Here's how the part is built. I have some questions about the finished solid (model axes, mm). Give positions to 0.01 mm unless a question says otherwise; leave off trailing zeros. Loops run counter-clockwise (first coordinate to the right, second up) from the corner with the lowest first, then second, coordinate; pieces in that order, holes last. Notation, with made-up numbers: (71, 60) - (93, 60) arc R22 cw to (93, 82) - close; hole circle Ø1 at (-33, 70.5). An arc over 180 degrees is marked (long way). Use a Markdown table: item, result.
from build123d import *
from OCP.BRepFilletAPI import BRepFilletAPI_MakeChamfer

# Parameters (mm, degrees)
SKETCH1_W                     = 2.54
SKETCH1_H                     = 2.54
MAIN_BODY_DEPTH               = 2.54
SKETCH3_W                     = 1.778
SKETCH3_H                     = 0.381
CUT_EXTRUDE1_DEPTH            = 5.399409051
CUT_EXTRUDE2_DEPTH            = 5.399409051
BODY_PATTERN_COUNT            = 3
BODY_PATTERN_PITCH            = 2.54
PIN_START                     = -5.54
SKETCH2_W                     = 0.64
SKETCH2_H                     = 0.64
PIN_DEPTH                     = 11.54
CHAMFER1_SIZE                 = 0.508
CHAMFER1_SIZE2                = 0.1905
CHAMFER2_SIZE                 = 0.1905
CHAMFER2_SIZE2                = 0.508
PIN_PATTERN_COUNT             = 3
PIN_PATTERN_PITCH             = 2.54
CHAMFER1_OF_PIN_PATTERN_SIZE  = 0.508
CHAMFER1_OF_PIN_PATTERN_SIZE2 = 0.1905
CHAMFER2_OF_PIN_PATTERN_SIZE2 = 0.1905
CHAMFER2_OF_PIN_PATTERN_SIZE  = 0.508


with BuildPart() as part:
    # Sketch1 → Main Body (new body)
    with BuildSketch(Plane(origin=(0, 0, 0), x_dir=(1, 0, 0), z_dir=(0, 1, 0))):
        with Locations((1.27, 1.27)):
            Rectangle(SKETCH1_W, SKETCH1_H)
    main_body = extrude(amount=MAIN_BODY_DEPTH)

    # Sketch3 → Cut-Extrude1 (cut, through all)
    with BuildSketch(Plane.ZY):
        with Locations((-1.27, 0.1905)):
            Rectangle(SKETCH3_W, SKETCH3_H)
    cut_extrude1 = extrude(amount=-CUT_EXTRUDE1_DEPTH, mode=Mode.SUBTRACT)

    # Sketch4 → Cut-Extrude2 (cut, through all)
    with BuildSketch(Plane(origin=(0, 2.54, 0), x_dir=(1, 0, 0), z_dir=(0, 1, 0))):
        Polygon((0.254, 2.54), (0, 2.54), (0, 2.032), align=None)
        Polygon((2.54, 2.54), (2.286, 2.54), (2.54, 2.032), align=None)
        Polygon((0.254, 0), (0, 0.508), (0, 0), align=None)
        Polygon((2.54, 0), (2.286, 0), (2.54, 0.508), align=None)
    cut_extrude2 = extrude(amount=-CUT_EXTRUDE2_DEPTH, mode=Mode.SUBTRACT)

    # Body Pattern: Main Body, Cut-Extrude1, Cut-Extrude2 ×3
    with Locations(*[(-i * BODY_PATTERN_PITCH, 0, 0) for i in range(1, BODY_PATTERN_COUNT)]):
        add(main_body)
        add(cut_extrude1, mode=Mode.SUBTRACT)
        add(cut_extrude2, mode=Mode.SUBTRACT)

    # Sketch2 → Pin (add)
    with BuildSketch(Plane(origin=(0, 2.54, 0), x_dir=(1, 0, 0), z_dir=(0, 1, 0)).offset(PIN_START)):
        with Locations((1.27, 1.27)):
            Rectangle(SKETCH2_W, SKETCH2_H)
    pin = extrude(amount=PIN_DEPTH)

    # Chamfer1: one chamfer whose edges measure the first distance from different faces: ONE call of the kernel's chamfer builder (chamfer() names one face for all edges)
    chamfer1_edges_1 = [part.edges().sort_by_distance(p)[0] for p in [
        (0.95, 8.54, -1.27),
    ]]
    chamfer1_side_1 = [part.faces().sort_by_distance(p)[0] for p in [
        (0.95, 5.54, -1.27),
    ]]
    chamfer1_edges_2 = [part.edges().sort_by_distance(p)[0] for p in [
        (1.27, 8.54, -0.95),
    ]]
    chamfer1_side_2 = [part.faces().sort_by_distance(p)[0] for p in [
        (1.27, 5.54, -0.95),
    ]]
    chamfer1_edges_3 = [part.edges().sort_by_distance(p)[0] for p in [
        (1.59, 8.54, -1.27),
    ]]
    chamfer1_side_3 = [part.faces().sort_by_distance(p)[0] for p in [
        (1.59, 5.54, -1.27),
    ]]
    chamfer1_edges_4 = [part.edges().sort_by_distance(p)[0] for p in [
        (1.27, 8.54, -1.59),
    ]]
    chamfer1_side_4 = [part.faces().sort_by_distance(p)[0] for p in [
        (1.27, 5.54, -1.59),
    ]]
    chamfer1 = BRepFilletAPI_MakeChamfer(part.part.solid().wrapped)
    for e in chamfer1_edges_1:
        chamfer1.Add(CHAMFER1_SIZE, CHAMFER1_SIZE2, e.wrapped, chamfer1_side_1[0].wrapped)  # the first distance lies on this face
    for e in chamfer1_edges_2:
        chamfer1.Add(CHAMFER1_SIZE, CHAMFER1_SIZE2, e.wrapped, chamfer1_side_2[0].wrapped)  # the first distance lies on this face
    for e in chamfer1_edges_3:
        chamfer1.Add(CHAMFER1_SIZE, CHAMFER1_SIZE2, e.wrapped, chamfer1_side_3[0].wrapped)  # the first distance lies on this face
    for e in chamfer1_edges_4:
        chamfer1.Add(CHAMFER1_SIZE, CHAMFER1_SIZE2, e.wrapped, chamfer1_side_4[0].wrapped)  # the first distance lies on this face
    add(Compound.cast(chamfer1.Shape()), mode=Mode.REPLACE)

    # Chamfer2
    chamfer2_edges = [part.edges().sort_by_distance(p)[0] for p in [
        (1.27, -3, -0.95),
        (1.59, -3, -1.27),
        (1.27, -3, -1.59),
        (0.95, -3, -1.27),
    ]]
    chamfer2_side = [part.faces().sort_by_distance(p)[0] for p in [
        (1.27, -3, -1.27),
    ]]
    chamfer(chamfer2_edges, length=CHAMFER2_SIZE, length2=CHAMFER2_SIZE2, reference=chamfer2_side[0])

    # Pin Pattern: Pin ×3
    with Locations(*[(-i * PIN_PATTERN_PITCH, 0, 0) for i in range(1, PIN_PATTERN_COUNT)]):
        add(pin)

    # Chamfer1 of Pin Pattern: one chamfer whose edges measure the first distance from different faces: ONE call of the kernel's chamfer builder (chamfer() names one face for all edges)
    chamfer1_of_pin_pattern_edges_1 = [part.edges().sort_by_distance(p)[0] for p in [
        (-1.59, 8.54, -1.27),
    ]]
    chamfer1_of_pin_pattern_side_1 = [part.faces().sort_by_distance(p)[0] for p in [
        (-1.59, 5.54, -1.27),
    ]]
    chamfer1_of_pin_pattern_edges_2 = [part.edges().sort_by_distance(p)[0] for p in [
        (-1.27, 8.54, -0.95),
    ]]
    chamfer1_of_pin_pattern_side_2 = [part.faces().sort_by_distance(p)[0] for p in [
        (-1.27, 5.54, -0.95),
    ]]
    chamfer1_of_pin_pattern_edges_3 = [part.edges().sort_by_distance(p)[0] for p in [
        (-0.95, 8.54, -1.27),
    ]]
    chamfer1_of_pin_pattern_side_3 = [part.faces().sort_by_distance(p)[0] for p in [
        (-0.95, 5.54, -1.27),
    ]]
    chamfer1_of_pin_pattern_edges_4 = [part.edges().sort_by_distance(p)[0] for p in [
        (-1.27, 8.54, -1.59),
    ]]
    chamfer1_of_pin_pattern_side_4 = [part.faces().sort_by_distance(p)[0] for p in [
        (-1.27, 5.54, -1.59),
    ]]
    chamfer1_of_pin_pattern_edges_5 = [part.edges().sort_by_distance(p)[0] for p in [
        (-4.13, 8.54, -1.27),
    ]]
    chamfer1_of_pin_pattern_side_5 = [part.faces().sort_by_distance(p)[0] for p in [
        (-4.13, 5.54, -1.27),
    ]]
    chamfer1_of_pin_pattern_edges_6 = [part.edges().sort_by_distance(p)[0] for p in [
        (-3.81, 8.54, -0.95),
    ]]
    chamfer1_of_pin_pattern_side_6 = [part.faces().sort_by_distance(p)[0] for p in [
        (-3.81, 5.54, -0.95),
    ]]
    chamfer1_of_pin_pattern_edges_7 = [part.edges().sort_by_distance(p)[0] for p in [
        (-3.49, 8.54, -1.27),
    ]]
    chamfer1_of_pin_pattern_side_7 = [part.faces().sort_by_distance(p)[0] for p in [
        (-3.49, 5.54, -1.27),
    ]]
    chamfer1_of_pin_pattern_edges_8 = [part.edges().sort_by_distance(p)[0] for p in [
        (-3.81, 8.54, -1.59),
    ]]
    chamfer1_of_pin_pattern_side_8 = [part.faces().sort_by_distance(p)[0] for p in [
        (-3.81, 5.54, -1.59),
    ]]
    chamfer1_of_pin_pattern = BRepFilletAPI_MakeChamfer(part.part.solid().wrapped)
    for e in chamfer1_of_pin_pattern_edges_1:
        chamfer1_of_pin_pattern.Add(CHAMFER1_OF_PIN_PATTERN_SIZE, CHAMFER1_OF_PIN_PATTERN_SIZE2, e.wrapped, chamfer1_of_pin_pattern_side_1[0].wrapped)  # the first distance lies on this face
    for e in chamfer1_of_pin_pattern_edges_2:
        chamfer1_of_pin_pattern.Add(CHAMFER1_OF_PIN_PATTERN_SIZE, CHAMFER1_OF_PIN_PATTERN_SIZE2, e.wrapped, chamfer1_of_pin_pattern_side_2[0].wrapped)  # the first distance lies on this face
    for e in chamfer1_of_pin_pattern_edges_3:
        chamfer1_of_pin_pattern.Add(CHAMFER1_OF_PIN_PATTERN_SIZE, CHAMFER1_OF_PIN_PATTERN_SIZE2, e.wrapped, chamfer1_of_pin_pattern_side_3[0].wrapped)  # the first distance lies on this face
    for e in chamfer1_of_pin_pattern_edges_4:
        chamfer1_of_pin_pattern.Add(CHAMFER1_OF_PIN_PATTERN_SIZE, CHAMFER1_OF_PIN_PATTERN_SIZE2, e.wrapped, chamfer1_of_pin_pattern_side_4[0].wrapped)  # the first distance lies on this face
    for e in chamfer1_of_pin_pattern_edges_5:
        chamfer1_of_pin_pattern.Add(CHAMFER1_OF_PIN_PATTERN_SIZE, CHAMFER1_OF_PIN_PATTERN_SIZE2, e.wrapped, chamfer1_of_pin_pattern_side_5[0].wrapped)  # the first distance lies on this face
    for e in chamfer1_of_pin_pattern_edges_6:
        chamfer1_of_pin_pattern.Add(CHAMFER1_OF_PIN_PATTERN_SIZE, CHAMFER1_OF_PIN_PATTERN_SIZE2, e.wrapped, chamfer1_of_pin_pattern_side_6[0].wrapped)  # the first distance lies on this face
    for e in chamfer1_of_pin_pattern_edges_7:
        chamfer1_of_pin_pattern.Add(CHAMFER1_OF_PIN_PATTERN_SIZE, CHAMFER1_OF_PIN_PATTERN_SIZE2, e.wrapped, chamfer1_of_pin_pattern_side_7[0].wrapped)  # the first distance lies on this face
    for e in chamfer1_of_pin_pattern_edges_8:
        chamfer1_of_pin_pattern.Add(CHAMFER1_OF_PIN_PATTERN_SIZE, CHAMFER1_OF_PIN_PATTERN_SIZE2, e.wrapped, chamfer1_of_pin_pattern_side_8[0].wrapped)  # the first distance lies on this face
    add(Compound.cast(chamfer1_of_pin_pattern.Shape()), mode=Mode.REPLACE)

    # Chamfer2 of Pin Pattern
    chamfer2_of_pin_pattern_edges = [part.edges().sort_by_distance(p)[0] for p in [
        (-1.27, -3, -0.95),
        (-0.95, -3, -1.27),
        (-1.27, -3, -1.59),
        (-1.59, -3, -1.27),
        (-3.81, -3, -0.95),
        (-3.49, -3, -1.27),
        (-3.81, -3, -1.59),
        (-4.13, -3, -1.27),
    ]]
    chamfer(chamfer2_of_pin_pattern_edges, length=CHAMFER2_OF_PIN_PATTERN_SIZE, length2=CHAMFER2_OF_PIN_PATTERN_SIZE2)


solid = part.part
(1) If I drill on line 1 (X direction, y = 6.75, z = -1.2); line 2 (Z direction, x = 1, y = 0.25); line 3 (Z direction, x = -1.5, y = 5), over which ranges is the centre line in solid material (lowest first)?
A:
| item | result |
|---|---|
| line 1 | -4.13 to -3.49, -1.59 to -0.95, 0.95 to 1.59 |
| line 2 | -2.54 to -2.16, -1.59 to -0.95, -0.38 to 0 |
| line 3 | -1.59 to -0.95 |
(2) We'd pull the mould along X, two halves only. Please class faces 1 (the face through (-5.08, 1, -1)), 2 (the face through (-1, 0.381, -2)), 3 (the face through (-1, 1, 0)): pulls with the +X half, pulls with the -X half, needs draft (parallel to the pull), parting line crosses it, or undercut.
A:
| item | result |
|---|---|
| face 1 | pulls with the -X half |
| face 2 | undercut |
| face 3 | needs draft |
(3) Suppose I cut it at B-B on z = -0.2. Write out the boundary of the cut face in (x, y), plus the area to 3 significant figures.
A:
| item | result |
|---|---|
| outline | (-4.93, 0) - (-2.69, 0) - (-2.69, 2.54) - (-4.93, 2.54) - close; (-2.39, 0) - (-0.15, 0) - (-0.15, 2.54) - (-2.39, 2.54) - close; (0.15, 0) - (2.39, 0) - (2.39, 2.54) - (0.15, 2.54) - close |
| area | 17.0 mm2 |
(4) Suppose I cut it at A-A on y = 5.75. Write out the boundary of the cut face in (x, z).
A:
| item | result |
|---|---|
| outline | (-4.13, -1.59) - (-3.49, -1.59) - (-3.49, -0.95) - (-4.13, -0.95) - close; (-1.59, -1.59) - (-0.95, -1.59) - (-0.95, -0.95) - (-1.59, -0.95) - close; (0.95, -1.59) - (1.59, -1.59) - (1.59, -0.95) - (0.95, -0.95) - close |
(5) Suppose I cut it at D-D on z = -0.8. Write out the boundary of the cut face in (x, y), plus the area to 3 significant figures.
A:
| item | result |
|---|---|
| outline | (-5.08, 0.38) - (2.54, 0.38) - (2.54, 2.54) - (-5.08, 2.54) - close |
| area | 16.5 mm2 |
(6) Will these pins go through, and if not, where does the flat tip stop? pin 1 (0.7 mm diameter, centred on x = -4, y = -0.5, fed in from -Z); pin 2 (0.7 mm diameter, centred on y = 6, z = -1.5, fed in from -X); pin 3 (1.5 mm diameter, centred on x = -2.5, z = -1, fed in from -Y).
A:
| item | result |
|---|---|
| pin 1 | z = -1.59 |
| pin 2 | x = -4.13 |
| pin 3 | y = 0 |
(7) Suppose I cut it at C-C on x = -0.5. Write out the boundary of the cut face in (y, z).
A:
| item | result |
|---|---|
| outline | (0, -2.54) - (2.54, -2.54) - (2.54, 0) - (0, 0) - (0, -0.38) - (0.38, -0.38) - (0.38, -2.16) - (0, -2.16) - close |
